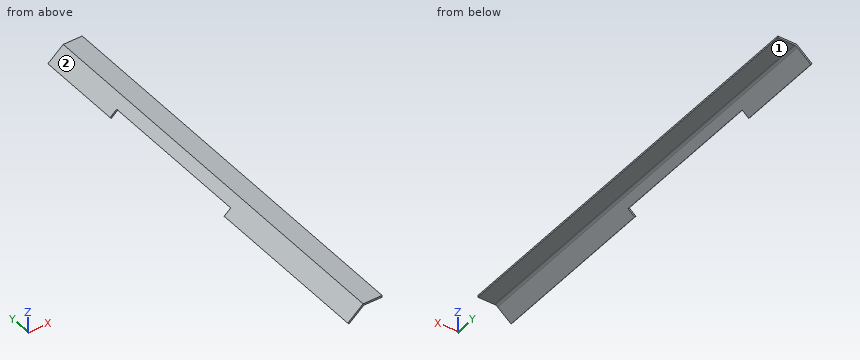
from build123d import *

# Parameters (mm, degrees)
EXTRUDE_START       = 40
EXTRUDE_1_DEPTH     = 460
SKETCH_2_W          = 14.817451962
SKETCH_2_H          = 174.961932368
CUT_EXTRUDE_1_DEPTH = 501.666670065


with BuildPart() as part:
    # Эскиз1 → Вытянуть1 (new body)
    with BuildSketch(Plane(origin=(0, 0, 0), x_dir=(1, 0, 0), z_dir=(0, 1, 0)).offset(EXTRUDE_START)):
        with BuildLine():
            Line((-20.508447565, 12.792651291), (-19.211965496, 14.315521688))
            Line((-19.211965496, 14.315521688), (-4.37520086, 1.680230584))
            ThreePointArc((-4.37520086, 1.680230584), (-2.860623355, 0.794693725), (-1.133379225, 0.48688167))
            Line((-1.133379225, 0.48688167), (17.122829042, 0.48688167))
            Line((17.122829042, 0.48688167), (17.122829042, -1.51311833))
            Line((17.122829042, -1.51311833), (-3.70464164, -1.51311833))
            Line((-3.70464164, -1.51311833), (-20.508447565, 12.792651291))
        make_face()
    extrude(amount=EXTRUDE_1_DEPTH)

    # Эскиз2 → Вырез-Вытянуть1 (cut, through all)
    with BuildSketch(Plane(origin=(-2.30361675, 0, 2.705868318), x_dir=(0.7614351985155554, 0, 0.6482410342315402), z_dir=(-0.6482410342315401, 0, 0.7614351985155553))):
        with Locations((-21.841147888, 317.116726633)):
            Rectangle(SKETCH_2_W, SKETCH_2_H)
    extrude(amount=-CUT_EXTRUDE_1_DEPTH, mode=Mode.SUBTRACT)


solid = part.part
Can you work these out from the model? Positions are in its coordinate system, mm. Face numbers are marked on the shaded views. A direction names the side the tool comes from. Coordinates: 2 decimals unless noted, no trailing zeros. Write each loop counter-clockwise with the first axis right and the second up, starting at its lowest first coordinate (ties: lowest second). Pieces come first, ordered by that corner, then holes. Notation, with made-up numbers: (-22, -20) -> (-15, -20) arc R17 cw to (-15, 4) -> close; hole circle Ø3 at (79, -37.75). An arc over 180 degrees is marked (long way). Write each question's results on one line, items separated by ' | '. Start each with the question number.
Item 1: I'm going to push flat-ended pins straight in: P1, Ø10, axis at x = -10, y = 350.5, coming from the +Z side; P2, Ø9, axis at x = 4.5, y = 372.5, coming from the -Z side. Where does each tip first touch, or does it pass through?
Item 2: If we section it at B-B, the plane y = 443.5: Write out the boundary of the cut face in (x, z).
Item 3: If we section it at C-C, the plane x = 5: Write out the boundary of the cut face in (y, z), and give its area (3 significant figures).
Item 4: On a 3-axis mill with a long thin cutter (end or side, diameter ignored), from which of +Z, -Z, +X, -X, +Y, -Y can I reach the whole of each face in a straight line? I mean the marked faces 1 and 2. Say none if no direction works.
Item 5: If we section it at A-A, the plane y = 263: Write out the boundary of the cut face in (x, z), and give its area (3 significant figures).
Item 6: Please list where these lines run through material, in increasing order: probe 1 along Z at (x, y) = (9, 68.5); probe 2 along Z at (x, y) = (-5, 467); probe 3 along X at (y, z) = (450, -3.25).
Answer block:
1) P1: z = 0.41 | P2: z = -0.49
2) outline: (-20.51, -12.79) -> (-19.21, -14.32) -> (-4.38, -1.68) arc R5 cw to (-1.13, -0.49) -> (17.12, -0.49) -> (17.12, 1.51) -> (-3.7, 1.51) -> close
3) outline: (40, -0.49) -> (500, -0.49) -> (500, 1.51) -> (40, 1.51) -> close | area: 920 mm²
4) face 1: -Z, +X, +Y, -Y | face 2: +Z, -X, +Y, -Y
5) outline: (-13.29, -6.65) -> (-12, -8.17) -> (-4.38, -1.68) arc R5 cw to (-1.13, -0.49) -> (17.12, -0.49) -> (17.12, 1.51) -> (-3.7, 1.51) -> close | area: 65.7 mm²
6) probe 1: -0.49 to 1.51 | probe 2: -2.21 to 0.41 | probe 3: -9.3 to -6.22
